Part print with two shaded views. Sizes in mm from the minimum x, y, z corner. Round coordinates to 2 decimals unless told otherwise and drop trailing zeros. Order: outer loops, then holes, each group sorted by start corner. A loop starts at its lowest first (then second) coordinate and runs counter-clockwise, first axis right, second up. Notation, with made-up numbers: M -30.75,67 L -11.75,67 A31 ccw -11.75,91 Z; hole C -38.75,54 d5. An arc over 180 degrees is marked long. Put each result on its own line as item: value.
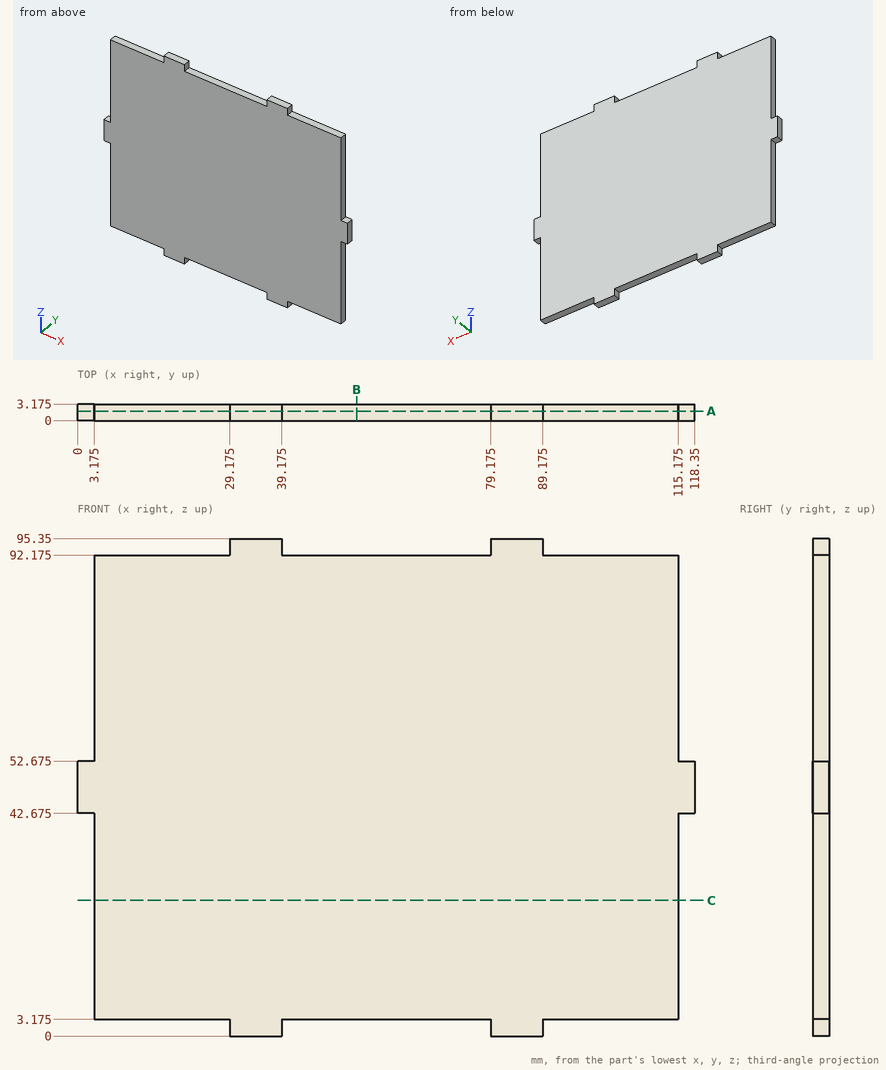
Item 1: Band-saw the part on B-B on x = 53.5. Give the cut face in (y, z) (3 decimals), and give its area (3 significant figures).
Answers below:
outline: M 0,3.175 L 3.175,3.175 L 3.175,92.175 L 0,92.175 Z
area: 283 mm²
Item 2: Pin check, flat tips, straight feed: P1, Ø1.6, axis at y = 1, z = 69.5, coming from the +X side (3 decimals); P2, Ø1.6, axis at y = 2.5, z = 1.5, coming from the +X side (3 decimals); P3, Ø1.6, axis at y = 1.5, z = 1.5, coming from the -X side (3 decimals). Stop position of each tip, or through.
Answers below:
P1: x = 115.175
P2: x = 89.175
P3: x = 29.175
Item 3: Band-saw the part on A-A on y = 1.8. Give the cut face in (x, z) (3 decimals), and give its area (3 significant figures).
Answers below:
outline: M 0,42.675 L 3.175,42.675 L 3.175,3.175 L 29.175,3.175 L 29.175,0 L 39.175,0 L 39.175,3.175 L 79.175,3.175 L 79.175,0 L 89.175,0 L 89.175,3.175 L 115.175,3.175 L 115.175,42.675 L 118.35,42.675 L 118.35,52.675 L 115.175,52.675 L 115.175,92.175 L 89.175,92.175 L 89.175,95.35 L 79.175,95.35 L 79.175,92.175 L 39.175,92.175 L 39.175,95.35 L 29.175,95.35 L 29.175,92.175 L 3.175,92.175 L 3.175,52.675 L 0,52.675 Z
area: 10,200 mm²
Item 4: Band-saw the part on C-C on z = 26. Give the cut face in (x, y) (3 decimals).
Answers below:
outline: M 3.175,0 L 115.175,0 L 115.175,3.175 L 3.175,3.175 Z
Item 5: Probe line 1 along Z through (x, y) = (39.5, 0.4) (3 decimals); line 2 along X through (y, z) = (0.15, 73) (3 decimals). List the from-to ranges inside material, lowest first. Write a range as [from, to].
Answers below:
line 1: [3.175, 92.175]
line 2: [3.175, 115.175]
